from build123d import *

# Parameters (mm, degrees)
F0_R     = 38.1
F0_R_2   = 33.02
F1_DEPTH = 25.4
F2_R     = 38.1
F3_DEPTH = 5.08
F4_R     = 73.66
F4_R_2   = 38.1
F5_DEPTH = 25.4
F7_DEPTH = 12.7
F8_R     = 2.5999948
F9_DEPTH = 22.0000068


with BuildPart() as f1:
    # F0 (on Top) → F1 (new body)
    with BuildSketch(Plane.XY):
        Circle(F0_R)
        Circle(F0_R_2, mode=Mode.SUBTRACT)
    extrude(amount=F1_DEPTH)

    # F2 (on face) → F3 (join)
    with BuildSketch(Plane.XY.offset(25.4)):
        Circle(F2_R)
    extrude(amount=F3_DEPTH)

    # F4 (on face) → F5 (join)
    with BuildSketch(Plane.XY.offset(30.48)):
        Circle(F4_R)
        Circle(F4_R_2, mode=Mode.SUBTRACT)
        Circle(F4_R_2)
    extrude(amount=F5_DEPTH)

    # F6 (on face) → F7 (cut)
    with BuildSketch(Plane.XY.offset(55.88)):
        with BuildLine():
            Line((-53.3851905178, -45.0449101829), (-6.0161168891, -2.0319541275))
            ThreePointArc((-6.0161168891, -2.0319541275), (-6.3123702779, -0.6902763759), (-6.3130838426, 0.6837195304))
            Line((-6.3130838426, 0.6837195304), (-61.8586847432, 32.4426512763))
            ThreePointArc((-61.8586847432, 32.4426512763), (-69.4360730566, -7.5930401345), (-53.3851905178, -45.0449101829))
        make_face()
        with BuildLine():
            ThreePointArc((-3.7915855726, 5.093758813), (-2.607121536, 5.7901137551), (-1.3005942796, 6.2153804807))
            Line((-1.3005942796, 6.2153804807), (11.7394100669, 68.8564358015))
            ThreePointArc((11.7394100669, 68.8564358015), (-28.6783368956, 63.6912513058), (-59.3371864733, 36.852690559))
            Line((-59.3371864733, 36.852690559), (-3.7915855726, 5.093758813))
        make_face()
        with BuildLine():
            ThreePointArc((3.672788134, 5.1800702044), (4.7010805558, 4.2687634752), (5.5092723722, 3.1575968597))
            Line((5.5092723722, 3.1575968597), (69.1140391724, 10.1129663932))
            ThreePointArc((69.1140391724, 10.1129663932), (51.7118861143, 46.9563982275), (16.7127924805, 67.8211255252))
            Line((16.7127924805, 67.8211255252), (3.672788134, 5.1800702044))
        make_face()
        with BuildLine():
            Line((69.6662602731, 5.0630701709), (6.0614934729, -1.8922993626))
            ThreePointArc((6.0614934729, -1.8922993626), (5.5125491033, -3.1518728375), (4.7055118589, -4.2638782986))
            Line((4.7055118589, -4.2638782986), (30.9754152415, -62.6062788434))
            ThreePointArc((30.9754152415, -62.6062788434), (59.3407754188, -36.8469113046), (69.85, 0))
            ThreePointArc((69.85, 0), (69.8040499544, 2.5332015239), (69.6662602731, 5.0630701709))
        make_face()
        with BuildLine():
            Line((26.3433242374, -64.6919760722), (0.0734208549, -6.3495755274))
            ThreePointArc((0.0734208549, -6.3495755274), (-1.2941378453, -6.216728017), (-2.601106109, -5.7928185722))
            Line((-2.601106109, -5.7928185722), (-49.9701797376, -48.8057746275))
            ThreePointArc((-49.9701797376, -48.8057746275), (-14.2355162987, -68.3840081869), (26.3433242374, -64.6919760722))
        make_face()
    extrude(amount=-F7_DEPTH, mode=Mode.SUBTRACT)

    # F8 (on face) → F9 (cut)
    with BuildSketch(Plane(origin=(0, 0, 25.4), x_dir=(1, 0, 0), z_dir=(0, 0, -1))):
        Circle(F8_R)
    extrude(amount=-F9_DEPTH, mode=Mode.SUBTRACT)


solid = f1.part
The model under review builds one solid part; all positions refer to its coordinate system, in mm. A direction names the side the tool comes from. Round coordinates to 2 decimals unless told otherwise and drop trailing zeros. Write each loop counter-clockwise with the first axis right and the second up, starting at its lowest first coordinate (ties: lowest second). Pieces come first, ordered by that corner, then holes. Notation, with made-up numbers: (4.25, 32) -> (52.25, 32) arc R8 ccw to (52.25, 36) -> close; hole circle Ø1 at (88, -8). An arc over 180 degrees is marked (long way). Answer as a JSON object with one key per item and string values.
1. We need section C-C on z = 37.5. State the section outline as (x, y) points, and give its area (3 significant figures).
Results found:
{"outline": "circle Ø147.32 at (0, 0); hole circle Ø5.2 at (0, 0)", "area": "17,000 mm^2"}
2. Clearance check with flat-ended pins moving along their axes: pin 1 (1 mm diameter, centred on x = -57.5, z = 33.5, fed in from -Y); pin 2 (2 mm diameter, centred on x = 14.5, y = -57, fed in from -Z); pin 3 (6 mm diameter, centred on y = 23.5, z = 27, fed in from -X). State where each tip first meets the part, or that it passes through.
Results found:
{"pin 1": "stops at y = -46.66", "pin 2": "stops at z = 30.48", "pin 3": "stops at x = -32.11"}
3. To check wall thickness, follow line 1 along Y through (x, z) = (0, 9); line 2 along Y through (x, z) = (33, 53); line 3 along Y through (x, z) = (0, 33). State the ranges of each line that lie inside material, in increasing order.
Results found:
{"line 1": "y = -38.1 to -33.02, 33.02 to 38.1", "line 2": "y = -65.85 to -61.56, 1.05 to 6.16, 61.56 to 65.85", "line 3": "y = -73.66 to -2.6, 2.6 to 73.66"}
4. We need section A-A on x = 45.5. State the section outline as (y, z) points.
Results found:
{"outline": "(-57.93, 30.48) -> (57.93, 30.48) -> (57.93, 55.88) -> (53, 55.88) -> (53, 43.18) -> (7.53, 43.18) -> (7.53, 55.88) -> (2.42, 55.88) -> (2.42, 43.18) -> (-53, 43.18) -> (-53, 55.88) -> (-57.93, 55.88) -> close"}
5. The part is to be moulded in two halves that separate along X. For faces 1 (the face through (0, 0, 55.88)), 2 (the face through (-14.802, -68.264, 49.619)), 3 (the face through (-12, -44, 43.18)), say which applies: pulls with the +X half, pulls with the -X half, needs draft (parallel to the pull), parting line crosses it, or undercut.
Results found:
{"face 1": "needs draft", "face 2": "undercut", "face 3": "undercut"}
6. We need section B-B on y = 29.5. State the section outline as (x, z) points.
Results found:
{"outline": "(-67.49, 30.48) -> (-24.11, 30.48) -> (-24.11, 0) -> (-14.83, 0) -> (-14.83, 25.4) -> (14.83, 25.4) -> (14.83, 0) -> (24.11, 0) -> (24.11, 30.48) -> (67.49, 30.48) -> (67.49, 55.88) -> (63.31, 55.88) -> (63.31, 43.18) -> (8.74, 43.18) -> (8.74, 55.88) -> (3.55, 55.88) -> (3.55, 43.18) -> (-46.48, 43.18) -> (-46.48, 55.88) -> (-56.71, 55.88) -> (-56.71, 43.18) -> (-63.31, 43.18) -> (-63.31, 55.88) -> (-67.49, 55.88) -> close"}
7. We need section D-D on x = -57. State the section outline as (y, z) points, and give its area (3 significant figures).
Results found:
{"outline": "(-46.66, 30.48) -> (46.66, 30.48) -> (46.66, 55.88) -> (40.37, 55.88) -> (40.37, 43.18) -> (35.52, 43.18) -> (35.52, 55.88) -> (29.66, 55.88) -> (29.66, 43.18) -> (-40.37, 43.18) -> (-40.37, 55.88) -> (-46.66, 55.88) -> close", "area": "1,420 mm^2"}
8. Machinability: for faces 4 (the face through (31.5, 9.9, 12.5)), 5 (the face through (52.099, 46.526, 49.619)), which of the approach directions +Z, -Z, +X, -X, +Y, -Y give a long, thin tool a straight path to every point of the face, cutting with its end or side? Answer none if there is none.
Results found:
{"face 4": "-Z", "face 5": "+Z"}
